Can you work these out from the model? Positions are in its coordinate system, mm. Face numbers are marked on the shaded views. A direction names the side the tool comes from. Round coordinates to 2 decimals unless told otherwise and drop trailing zeros. Order: outer loops, then holes, each group sorted by start corner. A loop starts at its lowest first (then second) coordinate and runs counter-clockwise, first axis right, second up. Notation, with made-up numbers: (58, -1.75) -> (64, -1.75) arc R22 cw to (64, 4.25) -> close; hole circle Ø11 at (85, -9). An arc over 180 degrees is marked (long way). One line per item, written item: value.
```python
from build123d import *

# Parameters (mm, degrees)
F0_R     = 11
F0_R_2   = 2.75
F1_DEPTH = 7
F0_R_3   = 12.5
F2_DEPTH = 1.5
F3_SIZE  = 0.5
F4_SIZE  = 1


with BuildPart() as f1:
    # F0 (on Top) → F1 (new body)
    with BuildSketch(Plane.XY):
        Circle(F0_R)
        Circle(F0_R_2, mode=Mode.SUBTRACT)
    extrude(amount=F1_DEPTH)

    # F0 (on Top) → F2 (join)
    with BuildSketch(Plane.XY):
        Circle(F0_R_3)
        Circle(F0_R, mode=Mode.SUBTRACT)
    extrude(amount=F2_DEPTH)

    # F3
    f3_edges = [f1.edges().sort_by_distance(p)[0] for p in [
        (-11, 0, 7),
    ]]
    chamfer(f3_edges, length=F3_SIZE)

    # F4
    f4_edges = [f1.edges().sort_by_distance(p)[0] for p in [
        (-2.75, 0, 0),
    ]]
    chamfer(f4_edges, length=F4_SIZE)


solid = f1.part
```
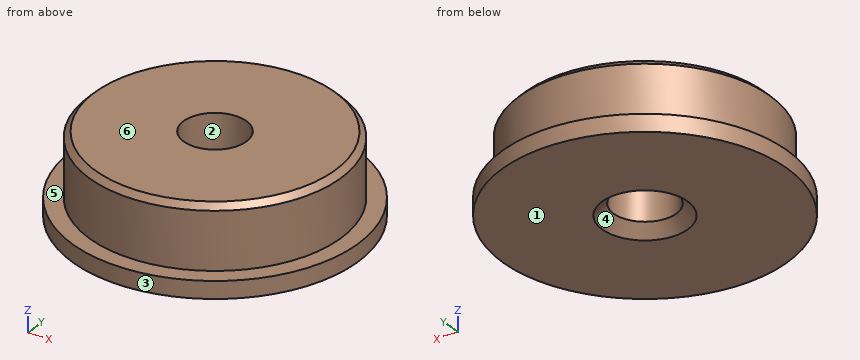
Q1. I want a section at A-A on y = 0. List the corners of the cut face in (x, z) for me.
Answers below:
outline: (-12.5, 0) -> (-3.75, 0) -> (-2.75, 1) -> (-2.75, 7) -> (-10.5, 7) -> (-11, 6.5) -> (-11, 1.5) -> (-12.5, 1.5) -> close; (2.75, 1) -> (3.75, 0) -> (12.5, 0) -> (12.5, 1.5) -> (11, 1.5) -> (11, 6.5) -> (10.5, 7) -> (2.75, 7) -> close
Q2. We'd pull the mould along X, two halves only. Please class the marked faces 1, 2, 3 and 4: released by +X, released by -X, zero draft, split by the parting line, or undercut.
Answers below:
face 1: zero draft
face 2: undercut
face 3: split by the parting line
face 4: undercut
Q3. I want a section at C-C on z = 2.75. List the corners of the cut face in (x, y) for me, plus the area to 3 significant figures.
Answers below:
outline: circle Ø22 at (0, 0); hole circle Ø5.5 at (0, 0)
area: 356 mm^2
Q4. Please list where these lines run through material, in increasing order: line 1 along Y through (x, z) = (0, 2.55); line 2 along Z through (x, y) = (-2.5, 11); line 3 along X through (y, z) = (-0.5, 5.5).
Answers below:
line 1: -11 to -2.75, 2.75 to 11
line 2: 0 to 1.5
line 3: -10.99 to -2.7, 2.7 to 10.99
Q5. On a 3-axis mill with a long thin cutter (end or side, diameter ignored), from which of +Z, -Z, +X, -X, +Y, -Y can I reach the whole of each face in a straight line? I mean the marked faces 5 and 6. Say none if no direction works.
Answers below:
face 5: +Z
face 6: +Z, +X, -X, +Y, -Y
Q6. Will these pins go through, and if not, where does the flat tip stop? pin 1 Ø5 at (x, y) = (-8, 7.5) entering from -Z; pin 2 Ø1 at (x, z) = (8, 5.5) entering from +Y.
Answers below:
pin 1: z = 0
pin 2: y = 8.05
